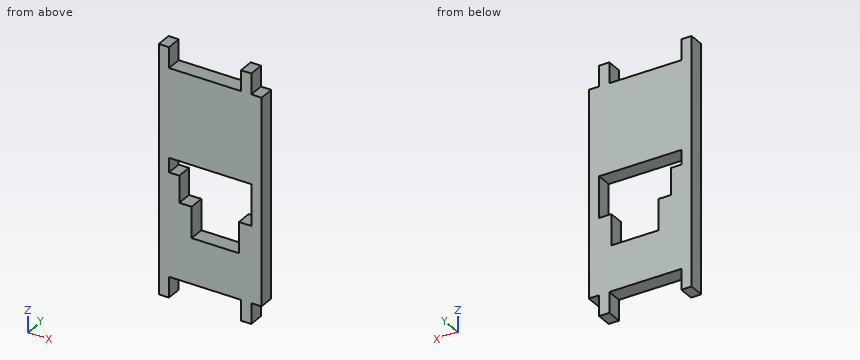
Autodesk Inventor part; units mm, degrees
ref_plane "YZ Plane" through (0, 0, 0) normal (1, 0, 0) x (0, 1, 0)
ref_plane "XZ Plane" through (0, 0, 0) normal (0, 1, 0) x (-1, 0, 0)
ref_plane "XY Plane" through (0, 0, 0) normal (0, 0, 1) x (1, 0, 0)
sketch "Sketch1" plane through (0, 0, 0) normal (0, 1, 0) x (-1, 0, 0)
  line L0 (50, 0) -> (50, 100)
  line L1 (0, 100) -> (0, 0)
  line L2 (34, 37) -> (34, 22)
  line L3 (34, 22) -> (22.5, 22)
  line L4 (11, 37) -> (11, 22)
  line L5 (11, 22) -> (22.5, 22)
  line L6 (34, 37) -> (40, 37)
  line L7 (11, 37) -> (5, 37)
  line L8 (40, 57) -> (5, 57)
  line L9 (5, 57) -> (5, 37)
  line L10 (40, 57) -> (45, 57)
  line L11 (45, 57) -> (45, 50)
  line L12 (45, 50) -> (40, 50)
  line L13 (45, 100) -> (45, 110)
  line L14 (45, 110) -> (50, 110)
  line L15 (50, 110) -> (50, 100)
  line L16 (5, 100) -> (5, 110)
  line L17 (45, 0) -> (45, -10)
  line L18 (45, -10) -> (50, -10)
  line L19 (50, -10) -> (50, 0)
  line L20 (5, 0) -> (5, -10)
  line L21 (40, 50) -> (40, 37)
  line L22 (5, 110) -> (10, 110)
  line L23 (10, 110) -> (10, 100)
  line L24 (5, 100) -> (5, 110)
  line L25 (5, -10) -> (10, -10)
  line L26 (10, -10) -> (10, 0)
  line L27 (5, 0) -> (5, -10)
  line L28 (0, 100) -> (5, 100)
  line L29 (10, 100) -> (45, 100)
  line L30 (0, 0) -> (5, 0)
  line L31 (45, 0) -> (10, 0)
  dimension "d1" = 100
  dimension "d10" = 5
  dimension "d11" = 5
  dimension "d12" = 5
  dimension "d13" = 10
  dimension "d16" = 5
  dimension "d17" = 10
  dimension "d22" = 5
  dimension "d23" = 10
extrude "Extrusion1" add sketch "Sketch1" along normal blind 7.5
properties part number "2P.01.01.02.JW.AilSerCage" material "Wood (Maple)"
Build history of the part. All positions in model axes, mm. Round coordinates to 2 decimals unless told otherwise and drop trailing zeros. Order: outer loops, then holes, each group sorted by start corner. A loop starts at its lowest first (then second) coordinate and runs counter-clockwise, first axis right, second up. Notation, with made-up numbers: (81.25, 55) -> (89.25, 55) arc R22 cw to (89.25, 83) -> close; hole circle Ø7 at (45, 88). An arc over 180 degrees is marked (long way). Answer in a Markdown table with one row per item.
1) Band-saw the part on C-C on y = 3.5. Give the cut face in (x, z).
Values:
| item | result |
|---|---|
| outline | (-50, -10) -> (-45, -10) -> (-45, 0) -> (-10, 0) -> (-10, -10) -> (-5, -10) -> (-5, 0) -> (0, 0) -> (0, 100) -> (-5, 100) -> (-5, 110) -> (-10, 110) -> (-10, 100) -> (-45, 100) -> (-45, 110) -> (-50, 110) -> close; hole (-45, 50) -> (-40, 50) -> (-40, 37) -> (-34, 37) -> (-34, 22) -> (-11, 22) -> (-11, 37) -> (-5, 37) -> (-5, 57) -> (-45, 57) -> close |
2) Band-saw the part on A-A on x = -36. Give the cut face in (y, z), and give its area (3 significant figures).
Values:
| item | result |
|---|---|
| outline | (0, 0) -> (7.5, 0) -> (7.5, 37) -> (0, 37) -> close; (0, 57) -> (7.5, 57) -> (7.5, 100) -> (0, 100) -> close |
| area | 600 mm2 |
3) Band-saw the part on B-B on z = 55.5. Give the cut face in (x, y).
Values:
| item | result |
|---|---|
| outline | (-50, 0) -> (-45, 0) -> (-45, 7.5) -> (-50, 7.5) -> close; (-5, 0) -> (0, 0) -> (0, 7.5) -> (-5, 7.5) -> close |
4) Wall check: L1, parallel to Z at x = -26, y = 3.5; L2, parallel to X at y = 5.75, z = -2; L3, parallel to X at y = 1, z = 55. Give the ranges that are in metal, low to high.
Values:
| item | result |
|---|---|
| L1 | 0 to 22, 57 to 100 |
| L2 | -50 to -45, -10 to -5 |
| L3 | -50 to -45, -5 to 0 |
5) Pin check, flat tips, straight feed: P1, Ø2, axis at y = 3.5, z = 41.5, coming from the +X side; P2, Ø4, axis at x = -41.5, y = 2.5, coming from the +Z side. Stop position of each tip, or through.
Values:
| item | result |
|---|---|
| P1 | x = 0 |
| P2 | z = 100 |
